Build history of the part. All positions in model axes, mm. Round coordinates to 2 decimals unless told otherwise and drop trailing zeros. Write each loop counter-clockwise with the first axis right and the second up, starting at its lowest first coordinate (ties: lowest second). Pieces come first, ordered by that corner, then holes. Notation, with made-up numbers: (-5, 48) -> (32, 48) arc R24 ccw to (32, 62) -> close; hole circle Ø7 at (-32.5, 68). An arc over 180 degrees is marked (long way). Answer in a Markdown table with one row per item.
```python
from build123d import *

# Parameters (mm, degrees)
SKETCH1_R           = 2.5000000000000004
BOSS_EXTRUDE1_DEPTH = 2
FILLET1_R           = 10
FILLET2_R           = 10
FILLET3_R           = 2
FILLET4_R           = 2


with BuildPart() as part:
    # Sketch1 → Boss-Extrude1 (new body)
    with BuildSketch(Plane(origin=(0, 0, 0), x_dir=(1, 0, 0), z_dir=(0, 1, 0))):
        with BuildLine():
            Line((4.734439187943633, 4.337505524576787), (-11.123424173439652, -8.60036927980545))
            Line((-11.123424173439652, -8.60036927980545), (-1.3192163601402593, -8.60036927980545))
            Line((-1.3192163601402593, -8.60036927980545), (10.29708605182919, 1.0617245936219641))
            Line((10.29708605182919, 1.0617245936219641), (13.693514413313048, 10.480195617492226))
            ThreePointArc((13.693514413313048, 10.480195617492226), (12.643820805599, 18.747230765158918), (7.611903426882685, 12.104525420451473))
            Line((7.611903426882685, 12.104525420451473), (4.734439187943633, 4.337505524576787))
        make_face()
        with Locations(Location((11.482625796556237, 14.39963072019455, 0), (0, 0, 270))):
            Circle(SKETCH1_R, mode=Mode.SUBTRACT)
    extrude(amount=BOSS_EXTRUDE1_DEPTH)

    # Fillet1
    fillet1_edges = [part.edges().sort_by_distance(p)[0] for p in [
        (10.29708605182919, 1, -1.0617245936219641),
    ]]
    fillet(fillet1_edges, radius=FILLET1_R)

    # Fillet2
    fillet2_edges = [part.edges().sort_by_distance(p)[0] for p in [
        (4.734439187943633, 1, -4.337505524576787),
    ]]
    fillet(fillet2_edges, radius=FILLET2_R)

    # Fillet3
    fillet3_edges = [part.edges().sort_by_distance(p)[0] for p in [
        (6.6461096923169105, 0, -9.49759844281185),
        (4.438286722207531, 0, -4.549211293465088),
        (12.456410034317898, 0, -7.049641368446211),
        (9.999920903343424, 0, -1.270100820961935),
        (-4.249333346620522, 0, 2.9920395518602865),
        (3.4439024153195033, 0, 4.638549149214148),
    ]]
    fillet(fillet3_edges, radius=FILLET3_R - 0.0001)  # a hair under: the kernel refuses the full size

    # Fillet4
    fillet4_edges = [part.edges().sort_by_distance(p)[0] for p in [
        (12.744313913733468, 3.2e-16, -18.719137994754206),
    ]]
    fillet(fillet4_edges, radius=FILLET4_R - 0.0001)  # a hair under: the kernel refuses the full size


solid = part.part
```
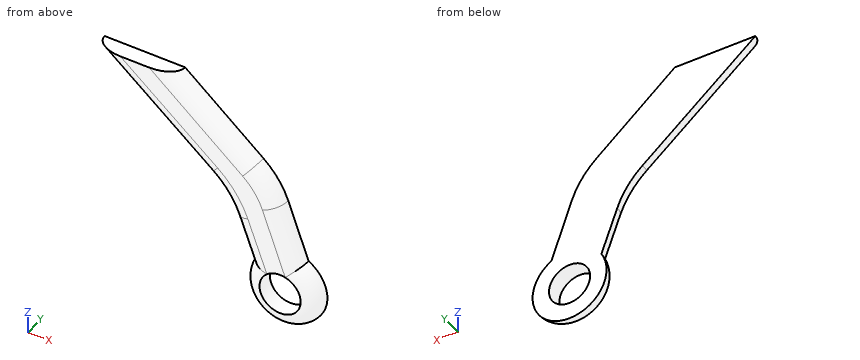
Q1. Saw through at A-A on y = 1.25. Write the cut outline in (x, z).
A:
| item | result |
|---|---|
| outline | (-10.89, 8.6) -> (2.72, -2.5) arc R10.15 cw to (5.82, -6.84) -> (7.77, -12.12) arc R4.35 ccw (long way) to (13.57, -10.58) -> (11.08, -3.67) arc R9.85 ccw to (8.11, 0.56) -> (-1.55, 8.6) -> close; hole circle Ø5 at (11.48, -14.4) |
Q2. Wall check: line 1 (X direction, y = 1.6, z = -13); line 2 (Y direction, x = -4.75, z = 5.5); line 3 (Y direction, x = 3.5, z = -2). Give the ranges that are in metal, low to high. Write a range as [from, to].
A:
| item | result |
|---|---|
| line 1 | [7.25, 9.41], [13.55, 15.72] |
| line 2 | [0.04, 2] |
| line 3 | [0.25, 2] |
Q3. Drop a flat-ended pin along its axis: P1, Ø1, axis at x = 6, y = 0.5, coming from the +Z side. Give the stop position or say it passes through.
A:
| item | result |
|---|---|
| P1 | z = 2.34 |
